Autodesk Inventor part; units mm, degrees
ref_plane "YZ Plane" through (0, 0, 0) normal (1, 0, 0) x (0, 1, 0)
ref_plane "XZ Plane" through (0, 0, 0) normal (0, 1, 0) x (-1, 0, 0)
ref_plane "XY Plane" through (0, 0, 0) normal (0, 0, 1) x (1, 0, 0)
sketch "Boceto1" plane through (0, 0, 0) normal (0, 1, 0) x (-1, 0, 0)
  line L0 (0, 0) -> (0, 16)
  line L1 (0, 16) -> (16, 16)
  line L2 (16, 16) -> (16, 0)
  line L3 (16, 0) -> (0, 0)
  line L4 (0, 16) -> (16, 0)
  circle A0 centre (8, 8) radius 11.3137
  circle A1 centre (16, 16) radius 1.5
  circle A2 centre (0, 16) radius 1.5
  circle A3 centre (0, 0) radius 1.5
  circle A4 centre (16, 0) radius 1.5
  circle A5 centre (8.1827, 7.8173) radius 16
  dimension "d0" = 16
  dimension "d1" = 16
  dimension "d2" = 3
  dimension "d5" = 360
  dimension "d7" = 32
extrude "Extrusión1" add sketch "Boceto1" along normal blind 2 contours A3 A0 A2 L0 | L0 A2 L4 A4 L3 A3 | L3 A4 A0 A3 | A2 L1 A1 L2 A4 L4 | A0 A1 L1 A2 | L2 A1 A0 A4 | A5
sketch "Boceto2" plane through (-8.1827, 2, 7.8173) normal (0, 1, 0) x (1, 0, 0)
  point P0 (8.1827, 7.8173)
sketch "Boceto3" plane through (-8.1827, 2, 7.8173) normal (0, 1, 0) x (1, 0, 0)
  circle A0 centre (0, 0) radius 6.5
  point P0 (8.1827, 7.8173)
  dimension "d10" = 13
extrude "Extrusión2" add sketch "Boceto3" along normal blind 15
sketch "Boceto4" plane through (-8.1827, 0, 7.8173) normal (0, -1, 0) x (1, 0, 0)
  circle A0 centre (8.1827, 8.1827) radius 1.5
  circle A1 centre (8.1827, 8.1827) radius 1.5
  circle A2 centre (8.1827, -7.8173) radius 1.5
  circle A3 centre (8.1827, -7.8173) radius 1.5
  circle A4 centre (-7.8173, -7.8173) radius 1.5
  circle A5 centre (-7.8173, -7.8173) radius 1.5
  circle A6 centre (-7.8173, 8.1827) radius 1.5
  circle A7 centre (-7.8173, 8.1827) radius 1.5
  point P0 (8.1827, -7.8173)
extrude "Extrusión3" add sketch "Boceto4" against normal blind 5
properties part number "brazo_2_contra"
Here's how the part is built. I have some questions about the finished solid (model axes, mm). A direction names the side the tool comes from. Give positions to 0.01 mm unless a question says otherwise; leave off trailing zeros. Loops run counter-clockwise (first coordinate to the right, second up) from the corner with the lowest first, then second, coordinate; pieces in that order, holes last. Notation, with made-up numbers: (80, 51.25) -> (124, 51.25) arc R26 ccw to (124, 85.25) -> close; hole circle Ø11 at (78, -21.5). An arc over 180 degrees is marked (long way). Answer as a JSON object with one key per item and string values. Group by question number.
Item 1: Imagine slicing it at B-B on z = 6. Write out the boundary of the cut face in (x, y).
Item 2: Imagine slicing it at A-A on y = 4. Write out the boundary of the cut face in (x, z), then the cut area to 3 significant figures.
Item 3: Will these pins go through, and if not, where does the flat tip stop? pin 1 (8 mm diameter, centred on x = 1, z = 20, fed in from +Y); pin 2 (5 mm diameter, centred on x = -5.5, y = 3, fed in from -Z); pin 3 (1.5 mm diameter, centred on x = -8.5, y = 8, fed in from -Z).
Item 4: Imagine slicing it at D-D on y = 14.5. Write out the boundary of the cut face in (x, z), then the cut area to 3 significant figures.
Item 5: On a 3-axis mill with a long thin cutter (end or side, diameter ignored), from which of +Z, -Z, +X, -X, +Y, -Y can I reach the whole of each face in a straight line? I mean faces 1 (the flat face through (0, 5, 16)), 2 (the cylindrical face through (-5.183, 9.395, 2.051)). Say none if no direction works.
Item 6: Imagine slicing it at C-C on x = -13.5. Write out the boundary of the cut face in (y, z).
Item 7: I need wall thicknesses on L1, parallel to Y at x = -2.5, z = 17.5; L2, parallel to X at y = 15, z = 9; L3, parallel to X at y = 1, z = -7. Which ranges of each line are inside material? Lowest first, please.
Item 8: Thinking about a two-plate mould opening in Z: for faces 3 (the cylindrical face through (-4.714, 0.986, 23.437)), 4 (the cylindrical face through (-17.5, 3.48, 16.07)), 5 (the flat face through (-8, 0, 8)), which applies, pulls with the +Z half, pulls with the -Z half, needs draft (parallel to the pull), parting line crosses it, or undercut?
Answer list:
{
 "1": {"outline": "(-24.08, 0) -> (7.71, 0) -> (7.71, 2) -> (-1.94, 2) -> (-1.94, 17) -> (-14.42, 17) -> (-14.42, 2) -> (-24.08, 2) -> close"},
 "2": {"outline": "circle Ø3 at (-16, 0); circle Ø3 at (-16, 16); circle Ø13 at (-8.18, 7.82); circle Ø3 at (0, 0); circle Ø3 at (0, 16)", "area": "161 mm2"},
 "3": {"pin 1": "stops at y = 5", "pin 2": "stops at z = -8.18", "pin 3": "stops at z = 1.32"},
 "4": {"outline": "circle Ø13 at (-8.18, 7.82)", "area": "133 mm2"},
 "5": {"face 1": "+Z, -Z, +X, -X, +Y", "face 2": "+Y"},
 "6": {"outline": "(0, -7.27) -> (2, -7.27) -> (2, 4.08) -> (17, 4.08) -> (17, 11.56) -> (2, 11.56) -> (2, 22.91) -> (0, 22.91) -> close"},
 "7": {"L1": "y = 0 to 2", "L2": "x = -14.57 to -1.79", "L3": "x = -14.22 to -2.15"},
 "8": {"face 3": "parting line crosses it", "face 4": "undercut", "face 5": "needs draft"}
}
